Geometry: final body of the model. Coordinates: model frame, mm. A direction names the side the tool comes from. Give positions to 0.01 mm unless a question says otherwise; leave off trailing zeros. Order: outer loops, then holes, each group sorted by start corner. A loop starts at its lowest first (then second) coordinate and runs counter-clockwise, first axis right, second up. Notation, with made-up numbers: (23.25, 38) - (33.25, 38) arc R21 ccw to (33.25, 77) - close; hole circle Ø7 at (59.25, 80.25). An arc over 180 degrees is marked (long way). Write item = value, one per line. Start each with the question number.
Autodesk Inventor part; units mm, degrees
ref_plane "YZ Plane" through (0, 0, 0) normal (1, 0, 0) x (0, 1, 0)
ref_plane "XZ Plane" through (0, 0, 0) normal (0, 1, 0) x (-1, 0, 0)
ref_plane "XY Plane" through (0, 0, 0) normal (0, 0, 1) x (1, 0, 0)
sketch "Sketch1" plane through (0, 0, 0) normal (0, 0, 1) x (1, 0, 0)
  line L0 (10, 5) -> (2, 5)
  arc A0 (2, 5) -> (0, 0) centre (7.25, 0) ccw
  arc A1 (12, 0) -> (10, 5) centre (4.75, 0) ccw
  line L1 (0, 0) -> (-5, 0)
  line L2 (-5, 0) -> (-5, 10)
  line L3 (-5, 10) -> (17, 10)
  line L4 (17, 10) -> (17, 0)
  line L5 (17, 0) -> (12, 0)
  dimension "d5" = 5
  dimension "d6" = 10
  dimension "d7" = 22
  dimension "d8" = 2
  dimension "d9" = 2
  dimension "d10" = 8
  dimension "d11" = 5
  dimension "d12" = 7.25
  dimension "d13" = 7.25
extrude "Extrusion1" add sketch "Sketch1" along normal blind 14
sketch "Sketch2" plane through (17, 0, 0) normal (1, 0, 0) x (0, 0, -1)
  line L0 (-14, 10) -> (-14, 0)
  line L1 (-14, 0) -> (0, 0)
  line L2 (0, 0) -> (0, 10)
  line L3 (0, 10) -> (-14, 10)
  line L4 (-14, 10) -> (-14, 0)
  dimension "d16" = 10
  dimension "d17" = 14
extrude "Extrusion2" add sketch "Sketch2" along normal blind 50
sketch "Sketch5" plane through (0, 0, 14) normal (0, 0, 1) x (1, 0, 0)
  line L0 (62, 0) -> (67, 0)
  line L1 (12, 0) -> (67, 0)
  arc A0 (12, 0) -> (10, 5) centre (4.75, 0) ccw
  arc A1 (2, 5) -> (0, 0) centre (7.25, 0) ccw
  line L2 (2, 5) -> (10, 5)
  arc A2 (62, 0) -> (60, 5) centre (54.75, 0) ccw
  arc A3 (52, 5) -> (50, 0) centre (57.25, 0) ccw
  line L3 (52, 5) -> (60, 5)
  line L4 (50, 0) -> (62, 0)
  dimension "d31" = 0
  dimension "d32" = 0
  dimension "d33" = 5
  dimension "d34" = 50
  dimension "d35" = 0
  dimension "d36" = 0
  dimension "d38" = 7.25
  dimension "d39" = 7.25
  dimension "d40" = 8
  dimension "d41" = 38
  dimension "d42" = 5
  dimension "d43" = 5
  dimension "d44" = 2
  dimension "d45" = 2
extrude "Extrusion3" cut sketch "Sketch5" against normal through all
properties part number "motorHolderTest1"
Q1. Section A-A, the plane y = 3.5. Return the cut outline in (x, z).
Q2. Section C-C, the plane x = 4. Return the cut outline in (y, z).
Q3. Section B-B, the plane z = 12.5. Return the cut outline in (x, y), then the cut area to 4 significant figures.
Q4. Contact query for flat-ended pins moving along their axis: pin 1 (2 mm diameter, centred on x = 46, y = 8.5, fed in from -Z); pin 2 (4 mm diameter, centred on x = 56.5, z = 8.5, fed in from -Y). Output: stop coordinate, or through.
Q5. Material intervals for line 1 along X through (y, z) = (0.5, 4.25); line 2 along X through (y, z) = (2.25, 10.5); line 3 along Y through (x, z) = (60, 2.25), sorted ascending. Write a range as from..to.
Q6. Set-up query: faces 1 (the flat face through (30, 5, 0)), 2 (the cylindrical face through (61.496, 2.657, 7.098)). Return all of +Z, -Z, +X, -X, +Y, -Y with unobstructed straight access to the full face (end or side cutting, diameter ignored); none if empty.
Q7. Pull-direction query (X, two-part tool) for faces 3 (the flat face through (67, 5, 7)), 4 (the cylindrical face through (50.533, 2.728, 7.098)), 5 (the flat face through (-5, 5, 7)), 6 (the flat face through (30, 10, 7)); classes: +X half, -X half, draft (parallel to the pull), parting line (faces both ways), or undercut.
The answers:
q1.outline = (-5, 0) - (0.9, 0) - (0.9, 14) - (-5, 14) - close; (11.1, 0) - (50.9, 0) - (50.9, 14) - (11.1, 14) - close; (61.1, 0) - (67, 0) - (67, 14) - (61.1, 14) - close
q2.outline = (5, 0) - (10, 0) - (10, 14) - (5, 14) - close
q3.outline = (-5, 0) - (0, 0) arc R7.25 cw to (2, 5) - (10, 5) arc R7.25 cw to (12, 0) - (50, 0) arc R7.25 cw to (52, 5) - (60, 5) arc R7.25 cw to (62, 0) - (67, 0) - (67, 10) - (-5, 10) - close
q3.area = 612.5 mm²
q4.pin_1 = 0
q4.pin_2 = 5
q5.line_1 = -5..0.02, 11.98..50.02, 61.98..67
q5.line_2 = -5..0.36, 11.64..50.36, 61.64..67
q5.line_3 = 5..10
q6.face_1 = -Z, +X, -X, +Y, -Y
q6.face_2 = +Z, -Z, -Y
q7.face_3 = +X half
q7.face_4 = undercut
q7.face_5 = -X half
q7.face_6 = draft
